from build123d import *

# Parameters (mm, degrees)
PAD_DEPTH    = 10
POCKET_DEPTH = 15
FILLET_R     = 9
FILLET001_R  = 5
FILLET002_R  = 2
FILLET003_R  = 1


with BuildPart() as part:
    # Sketch → Pad (new body, symmetric)
    with BuildSketch(Plane.YZ):
        with BuildLine():
            ThreePointArc((32.5, -1e-06), (1e-06, 32.5), (-32.5, 1e-06))
            Line((-32.5, -20), (-32.5, 1e-06))
            Line((-16.5, -20), (-32.5, -20))
            Line((-16.5, -20), (-16.5, 0))
            ThreePointArc((16.5, 5e-06), (-3e-06, 16.5), (-16.5, 0))
            Line((16.5, 5e-06), (16.5, -20))
            Line((32.5, -20), (16.5, -20))
            Line((32.5, -1e-06), (32.5, -20))
        make_face()
    extrude(amount=PAD_DEPTH, both=True)

    # Sketch001 → Pocket (cut)
    with BuildSketch(Plane.YZ.offset(10)):
        with BuildLine():
            Line((16.5, -20), (16.5, 5e-06))
            ThreePointArc((16.5, 5e-06), (-3e-06, 16.5), (-16.5, 0))
            Line((-16.5, 0), (-16.5, -20))
            Line((-28.5, -20), (-16.5, -20))
            Line((-28.5, 0), (-28.5, -20))
            ThreePointArc((28.5, 0), (0, 28.5), (-28.5, 0))
            Line((28.5, -20), (28.5, 0))
            Line((16.5, -20), (28.5, -20))
        make_face()
    extrude(amount=-POCKET_DEPTH, mode=Mode.SUBTRACT)

    # Fillet
    fillet_edges = [part.edges().sort_by_distance(p)[0] for p in [
        (-5, 0, 28.5),
    ]]
    fillet(fillet_edges, radius=FILLET_R)

    # Fillet001
    fillet001_edges = [part.edges().sort_by_distance(p)[0] for p in [
        (-10, 1e-06, 32.5),
    ]]
    fillet(fillet001_edges, radius=FILLET001_R)

    # Fillet002
    fillet002_edges = [part.edges().sort_by_distance(p)[0] for p in [
        (-8.535534, 31.035534, -20),
        (-8.535534, -31.035534, -20),
    ]]
    fillet(fillet002_edges, radius=FILLET002_R)

    # Fillet003
    fillet003_edges = [part.edges().sort_by_distance(p)[0] for p in [
        (-10, -3e-06, 16.5),
    ]]
    fillet(fillet003_edges, radius=FILLET003_R)


solid = part.part
Verification items for the finished model (mm, model axes). A direction names the side the tool comes from. Coordinates: 2 decimals unless noted, no trailing zeros. Write each loop counter-clockwise with the first axis right and the second up, starting at its lowest first coordinate (ties: lowest second). Pieces come first, ordered by that corner, then holes. Notation, with made-up numbers: (-31, 77.5) -> (-4, 77.5) arc R24 cw to (-4, 102.5) -> close; hole circle Ø8 at (54, 76). An arc over 180 degrees is marked (long way). One line per item, written item: value. Start each with the question number.
Q1. Cross-section at A-A on z = -7. Enter the section's corners in (x, y), and give its area (3 significant figures).
Q2. Cross-section at C-C on x = 1.75. Enter the section's corners in (y, z), and give its area (3 significant figures).
Q3. Go/stop test with flat-tipped pins: P1, Ø3, axis at x = -7, z = -12, coming from the +Y side; P2, Ø4, axis at x = 1, y = -4, coming from the +Z side; P3, Ø5, axis at x = -0.5, z = 11, coming from the +Y side. Record where each tip stops, or that it passes through.
Q4. Cross-section at B-B on x = 5.5. Enter the section's corners in (y, z), and give its area (3 significant figures).
Q5. Thickness scan on L1, parallel to Y at x = 7, z = -3.5; L2, parallel to Y at x = 1, z = -12.5; L3, parallel to X at y = -16.5, z = 8. Record the ranges inside material, lowest first. Write a range as from..to.
Q6. Mould release check, pull along Y, two halves, no side actions. Record for faces 4 (the cylindrical face through (2.6, -31.9, -19.43)), 5 (the flat face through (10, -7, 28)), 6 (the flat face through (-7, 16.5, -9)): pulls with the +Y half, pulls with the -Y half, needs draft (parallel to the pull), parting line crosses it, or undercut.
Q7. Access from +Z, -Z, +X, -X, +Y, -Y to the whole of each face (thin tool, end or side, straight path). Record for faces 1 (the flat face through (-5, 6, 16)), 2 (the flat face through (-7, -16.5, -10)), 3 (the cylindrical face through (-9.4, -22.57, -19.43)).
Checked values:
1. outline: (-10, -27.5) arc R5 ccw to (-5, -32.5) -> (10, -32.5) -> (10, -28.5) -> (4, -28.5) arc R9 cw to (-5, -19.5) -> (-5, -16.5) -> (-9, -16.5) arc R1 ccw to (-10, -17.5) -> close; (-10, 17.5) arc R1 ccw to (-9, 16.5) -> (-5, 16.5) -> (-5, 19.5) arc R9 cw to (4, 28.5) -> (10, 28.5) -> (10, 32.5) -> (-5, 32.5) arc R5 ccw to (-10, 27.5) -> close
1. area: 304 mm²
2. outline: (-32.5, -18) arc R2 ccw to (-30.5, -20) -> (-28.21, -20) -> (-28.21, 0) arc R28.21 cw to (28.21, 0) -> (28.21, -20) -> (30.5, -20) arc R2 ccw to (32.5, -18) -> (32.5, 0) arc R32.5 ccw to (-32.5, 0) -> close
2. area: 578 mm²
3. P1: stops at y = 32.47
3. P2: stops at z = 32.44
3. P3: stops at y = 31.37
4. outline: (-32.5, -18) arc R2 ccw to (-30.5, -20) -> (-28.5, -20) -> (-28.5, 0) arc R28.5 cw to (28.5, 0) -> (28.5, -20) -> (30.5, -20) arc R2 ccw to (32.5, -18) -> (32.5, 0) arc R32.5 ccw to (-32.5, 0) -> close
4. area: 542 mm²
5. L1: y = -32.5..-28.5, 28.5..32.5
5. L2: y = -32.5..-27.99, 27.99..32.5
5. L3: x = -10..-5
6. face 4: pulls with the -Y half
6. face 5: needs draft
6. face 6: undercut
7. face 1: -Z, +X
7. face 2: -Z, +X, -X
7. face 3: -Z, -X, +Y, -Y
